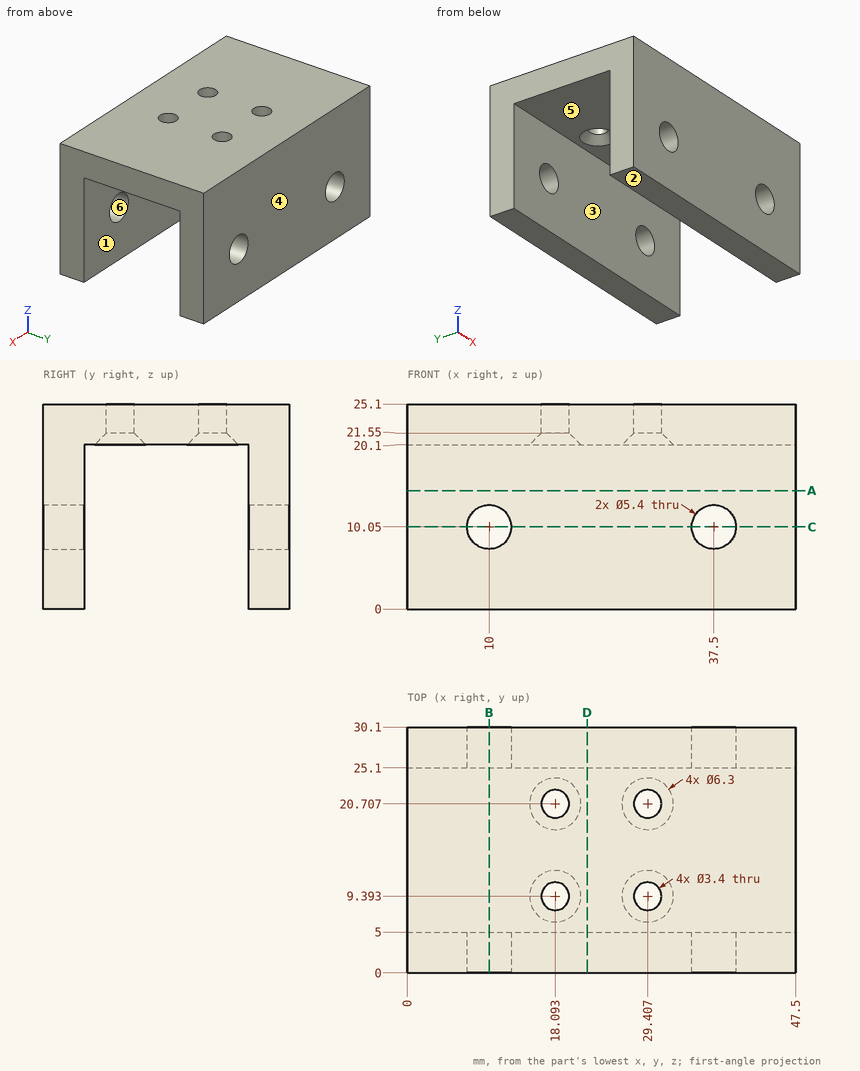
Source: three-view drawing plus pictorial views. Frame: mm from the lowest corner of the part. A direction names the side the tool comes from. Round coordinates to 2 decimals unless told otherwise and drop trailing zeros. Loops run counter-clockwise (first coordinate to the right, second up) from the corner with the lowest first, then second, coordinate; pieces in that order, holes last.
Item 1: Section A-A, the plane z = 14.5. Output: boundary loops of the cut face in (x, y), plus the area to 3 significant figures.
Checked values:
outline: (0, 0) - (47.5, 0) - (47.5, 5) - (0, 5) - close; (0, 25.1) - (47.5, 25.1) - (47.5, 30.1) - (0, 30.1) - close
area: 475 mm2
Item 2: Section B-B, the plane x = 10. Output: boundary loops of the cut face in (y, z).
Checked values:
outline: (0, 0) - (5, 0) - (5, 7.35) - (0, 7.35) - close; (0, 12.75) - (5, 12.75) - (5, 20.1) - (25.1, 20.1) - (25.1, 12.75) - (30.1, 12.75) - (30.1, 25.1) - (0, 25.1) - close; (25.1, 0) - (30.1, 0) - (30.1, 7.35) - (25.1, 7.35) - close
Item 3: Line query: L1, parallel to X at y = 27.95, z = 10.05; L2, parallel to Y at x = 7, z = 19.25; L3, parallel to Z at x = 10, y = 28.85. Output: solid intervals per line, ascending.
Checked values:
L1: x = 0 to 7.3, 12.7 to 34.8, 40.2 to 47.5
L2: y = 0 to 5, 25.1 to 30.1
L3: z = 0 to 7.35, 12.75 to 25.1
Item 4: Reachability of the marked faces 1 and 2 from +Z, -Z, +X, -X, +Y, -Y: full face, straight path, thin tool, end or side. Return the list, or none.
Checked values:
face 1: -Z, +X, -X
face 2: -Z, +X, -X, +Y, -Y
Item 5: Contact query for flat-ended pins moving along their axis: P1, Ø4.5, axis at x = 29.41, y = 9.39, coming from the -Z side (1 decimal); P2, Ø5, axis at x = 22, y = 21.5, coming from the -Z side; P3, Ø3, axis at x = 18, y = 9.5, coming from the +Z side. Output: stop coordinate, or through.
Checked values:
P1: stops at z = 21
P2: stops at z = 20.1
P3: passes through
Item 6: Section C-C, the plane z = 10.05. Output: boundary loops of the cut face in (x, y), plus the area to 3 significant figures.
Checked values:
outline: (0, 0) - (7.3, 0) - (7.3, 5) - (0, 5) - close; (0, 25.1) - (7.3, 25.1) - (7.3, 30.1) - (0, 30.1) - close; (12.7, 0) - (34.8, 0) - (34.8, 5) - (12.7, 5) - close; (12.7, 25.1) - (34.8, 25.1) - (34.8, 30.1) - (12.7, 30.1) - close; (40.2, 0) - (47.5, 0) - (47.5, 5) - (40.2, 5) - close; (40.2, 25.1) - (47.5, 25.1) - (47.5, 30.1) - (40.2, 30.1) - close
area: 367 mm2
Item 7: Section D-D, the plane x = 22. Output: boundary loops of the cut face in (y, z), plus the area to 4 significant figures.
Checked values:
outline: (0, 0) - (5, 0) - (5, 20.1) - (25.1, 20.1) - (25.1, 0) - (30.1, 0) - (30.1, 25.1) - (0, 25.1) - close
area: 351.5 mm2
Item 8: Mould query, pull axis Y, two halves, no side actions, for the marked faces 3, 4, 5 and 6. Classes: released by +Y, released by -Y, zero draft, split by the parting line, or undercut.
Checked values:
face 3: undercut
face 4: released by +Y
face 5: undercut
face 6: zero draft
